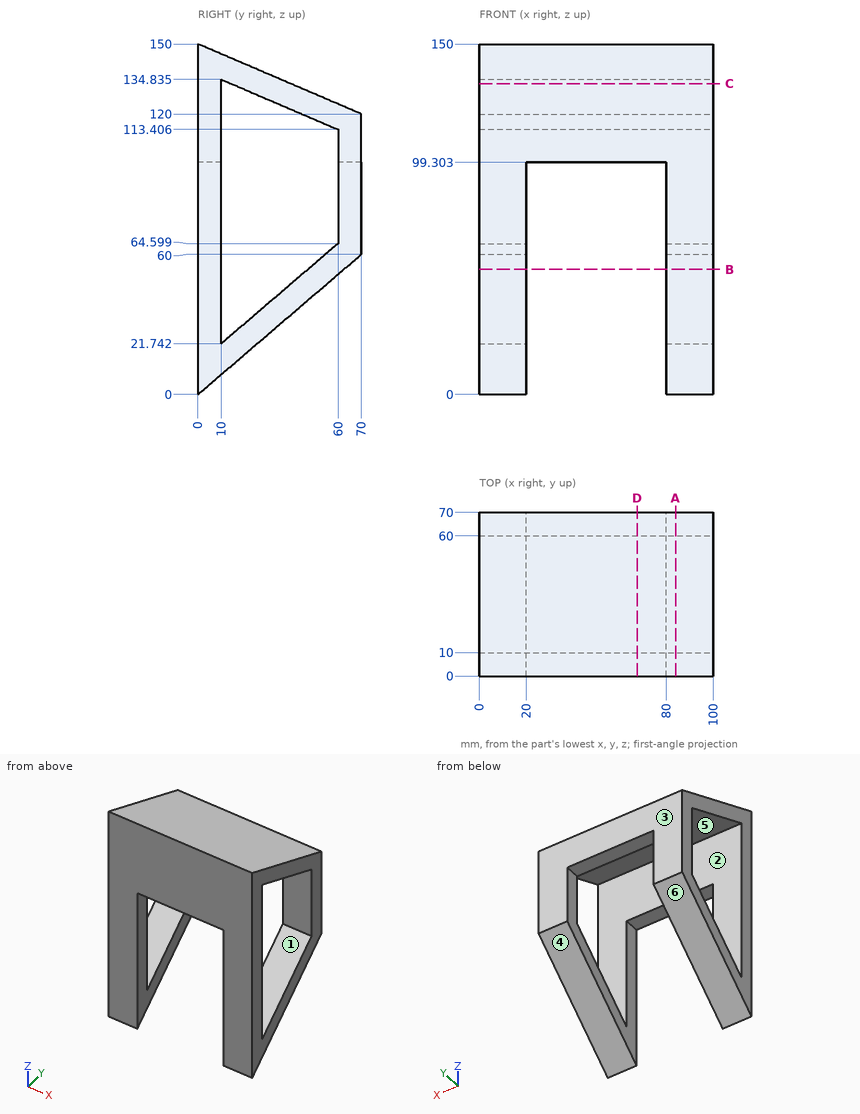
Drawing for the job (mm, zero at the part's lowest x, y, z). A direction names the side the tool comes from. Round coordinates to 2 decimals unless told otherwise and drop trailing zeros. Write each loop counter-clockwise with the first axis right and the second up, starting at its lowest first coordinate (ties: lowest second). Pieces come first, ordered by that corner, then holes. Notation, with made-up numbers: M 49,52 L 96,52 A32 cw 96,85 Z; hole C 42.25,39.5 d5. An arc over 180 degrees is marked long. One line per question, with ' | ' between items.
1. Cut at C-C on z = 133. Write the cut outline in (x, y), and give its area (3 significant figures).
Working result:
outline: M 0,0 L 100,0 L 100,10 L 0,10 Z; M 0,14.28 L 100,14.28 L 100,39.67 L 0,39.67 Z | area: 3,540 mm2
2. Probe L1, parallel to Y at x = 82.5, z = 98; L2, parallel to X at y = 62, z = 76; L3, parallel to Y at x = 14.5, z = 117 (1 decimal). List the from-to ranges inside material, lowest first. Write a range as from..to.
Working result:
L1: 0..10, 60..70 | L2: 0..20, 80..100 | L3: 0..10, 51.6..70
3. Which spindle directions (+Z, -Z, +X, -X, +Y, -Y) get a long thin tool onto all of the face, cutting with end or side? Do the marked faces 5 and 6. Say none if no direction does.
Working result:
face 5: +X, -X | face 6: -Z, +X, -X, +Y
4. Cut at D-D on x = 67.5. Write the cut outline in (y, z) (1 decimal), and give its area (3 significant figures).
Working result:
outline: M 0,99.3 L 10,99.3 L 10,134.8 L 60,113.4 L 60,99.3 L 70,99.3 L 70,120 L 0,150 Z | area: 1,260 mm2
5. Mould opens along Z. For the marked faces 1, 2, 3 and 4 say: pulls with the +Z half, pulls with the -Z half, needs draft (parallel to the pull), parting line crosses it, or undercut.
Working result:
face 1: undercut | face 2: undercut | face 3: needs draft | face 4: pulls with the -Z half
6. Cut at B-B on z = 53.5. Write the cut outline in (x, y), and give its area (3 significant figures).
Working result:
outline: M 0,0 L 20,0 L 20,10 L 0,10 Z; M 0,47.05 L 20,47.05 L 20,62.42 L 0,62.42 Z; M 80,0 L 100,0 L 100,10 L 80,10 Z; M 80,47.05 L 100,47.05 L 100,62.42 L 80,62.42 Z | area: 1,010 mm2
7. Pin check, flat tips, straight feed: pin 1 Ø5 at (x, z) = (84.5, 107.5) entering from -Y; pin 2 Ø12 at (x, y) = (44.5, 30.5) entering from -Z; pin 3 Ø12 at (x, y) = (62.5, 17) entering from +Z (1 decimal); pin 4 Ø5 at (x, y) = (40.5, 63.5) entering from -Z. Stop position of each tip, or through.
Working result:
pin 1: y = 0 | pin 2: z = 123.48 | pin 3: z = 145.3 | pin 4: z = 99.3
8. Cut at A-A on x = 84. Write the cut outline in (y, z) (1 decimal), and give its area (3 significant figures).
Working result:
outline: M 0,0 L 70,60 L 70,120 L 0,150 Z; hole M 10,21.7 L 60,64.6 L 60,113.4 L 10,134.8 Z | area: 3,300 mm2
